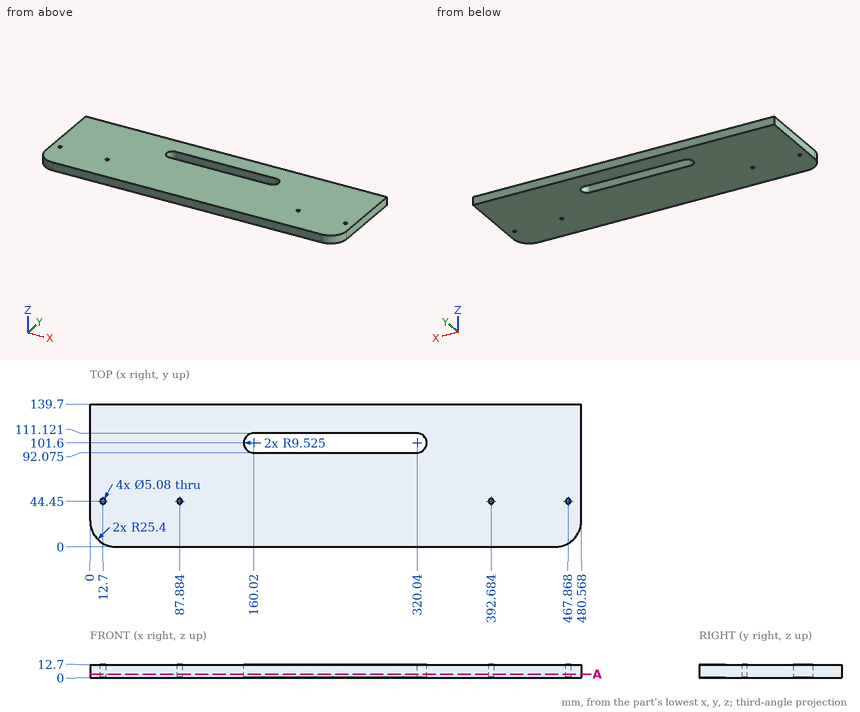
Can you work these out from the drawing? Everything is in mm from the part's minimum corner. Give positions to 0.01 mm unless a question says otherwise; leave off trailing zeros. Write each question's results on one line, items separated by ' | '.
Item 1: Suppose I cut it at A-A on z = 3.5. Give the number of separate pieces and of enclosed holes in the cut face, plus the area to 3 significant figures.
Output:
separate pieces: 1 | enclosed holes: 5 | area: 63,400 mm^2
Item 2: If I drill on L1, parallel to Y at x = 215, z = 9.25; L2, parallel to X at y = 16.5, z = 10; L3, parallel to Y at x = 12.7, z = 6.75, over which ranges is the centre line in solid material (lowest first)?
Output:
L1: y = 0 to 92.08, 111.12 to 139.7 | L2: x = 1.61 to 478.96 | L3: y = 3.4 to 41.91, 46.99 to 139.7
Item 3: For pin 1 Ø3 at (x, y) = (467.868, 44.45) entering from +Z, with a flat end and sliding along its axis, tell me the tip position at first contact or that it passes through.
Output:
pin 1: passes through
